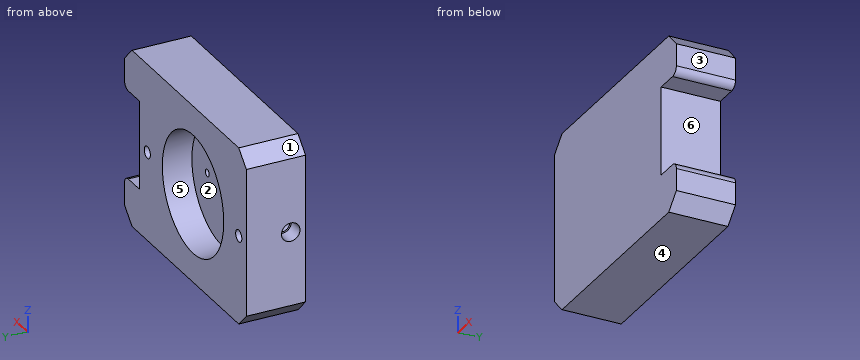
```python
from build123d import *

# Parameters (mm, degrees)
BOX_BODY_DEPTH                 = 25.4
SKETCH3_R                      = 25.5905
SAMPLE_HOLE_DEPTH              = 12.7
CUTOUT_EDGE_FILLET_R           = 3.175
BOX_EDGE_CHAMFER_SIZE          = 6.35
BOX_CLAMP_THREADED_HOLES_D     = 5.1054
BOX_CLAMP_THREADED_HOLES_DEPTH = 12.7
BOX_CLAMP_THREADED_HOLES_TIP   = 1.533816902
SKETCH10_R                     = 1.5875
CUT_EXTRUDE2_DEPTH             = 63.5
CUT_EXTRUDE3_REACH             = 14.7
FLUID_HOLES_R                  = 1.5875


with BuildPart() as part:
    # Sketch1 → box body (new body)
    with BuildSketch(Plane(origin=(0, 0, 0), x_dir=(1, 0, 0), z_dir=(0, 1, 0))):
        Polygon((-50.8, 38.1), (50.8, 38.1), (50.8, 19.05), (38.1, 19.05), (38.1, -19.05), (50.8, -19.05), (50.8, -38.1), (-50.8, -38.1), align=None)
    extrude(amount=BOX_BODY_DEPTH)

    # Sketch3 → sample hole (cut)
    with BuildSketch(Plane(origin=(0, 25.4, 0), x_dir=(1, 0, 0), z_dir=(0, 1, 0))):
        with Locations((-6.35, 0)):
            Circle(SKETCH3_R)
    extrude(amount=-SAMPLE_HOLE_DEPTH, mode=Mode.SUBTRACT)

    # cutout edge fillet
    cutout_edge_fillet_edges = [part.edges().sort_by_distance(p)[0] for p in [
        (50.8, 12.7, -19.05),
        (50.8, 12.7, 19.05),
    ]]
    fillet(cutout_edge_fillet_edges, radius=CUTOUT_EDGE_FILLET_R)

    # box edge chamfer
    box_edge_chamfer_edges = [part.edges().sort_by_distance(p)[0] for p in [
        (50.8, 12.7, 38.1),
        (-50.8, 12.7, 38.1),
        (-50.8, 12.7, -38.1),
        (50.8, 12.7, -38.1),
    ]]
    chamfer(box_edge_chamfer_edges, length=BOX_EDGE_CHAMFER_SIZE)

    # box clamp threaded holes
    with Locations(Plane(origin=(0, 25.4, 0), x_dir=(1, 0, 0), z_dir=(0, 1, 0))):
        with Locations((-44.45, 0), (31.75, 0)):
            Hole(BOX_CLAMP_THREADED_HOLES_D / 2, depth=BOX_CLAMP_THREADED_HOLES_DEPTH)
            with Locations((0, 0, -(BOX_CLAMP_THREADED_HOLES_DEPTH + BOX_CLAMP_THREADED_HOLES_TIP / 2))):  # 118° drill point
                Cone(0, BOX_CLAMP_THREADED_HOLES_D / 2, BOX_CLAMP_THREADED_HOLES_TIP, mode=Mode.SUBTRACT)

    # Sketch10 → Cut-Extrude2 (cut)
    with BuildSketch(Plane.ZY.offset(50.8)):
        with Locations((0, 6.35)):
            Circle(SKETCH10_R)
    extrude(amount=-CUT_EXTRUDE2_DEPTH, mode=Mode.SUBTRACT)

    # fluid holes → Cut-Extrude3 (cut, up to next)
    with BuildSketch(Plane(origin=(0, 12.7, 0), x_dir=(1, 0, 0), z_dir=(0, 1, 0)), mode=Mode.PRIVATE) as cut_extrude3_sk1:
        with Locations((-19.14525, 0)):
            Circle(FLUID_HOLES_R)
    cut_extrude3_tool1 = extrude(cut_extrude3_sk1.sketch, amount=-CUT_EXTRUDE3_REACH, mode=Mode.PRIVATE) & part.part
    add(cut_extrude3_tool1.solids().sort_by_distance((-19.14525, 12.7, 0))[0], mode=Mode.SUBTRACT)
    # fluid holes → Cut-Extrude3 (cut, up to next)
    with BuildSketch(Plane(origin=(0, 12.7, 0), x_dir=(1, 0, 0), z_dir=(0, 1, 0)), mode=Mode.PRIVATE) as cut_extrude3_sk2:
        with Locations((6.44525, 0)):
            Circle(FLUID_HOLES_R)
    cut_extrude3_tool2 = extrude(cut_extrude3_sk2.sketch, amount=-CUT_EXTRUDE3_REACH, mode=Mode.PRIVATE) & part.part
    add(cut_extrude3_tool2.solids().sort_by_distance((6.44525, 12.7, 0))[0], mode=Mode.SUBTRACT)

    # Sketch15 → 1/16 NPT Tapped Hole2 (revolve, cut)
    with BuildSketch(Plane(origin=(-50.8, 6.35, 0), x_dir=(0, 0, 1), z_dir=(0, 1, 0))):
        Polygon((0, 0), (0, 13.530685027), (3.0734, 11.684), (3.0734, 6.858), (3.762574096, 6.858), (3.9679118, 0), align=None)
    revolve(axis=Axis((-57.15, 6.35, 0), (1, 0, 0)), mode=Mode.SUBTRACT)


solid = part.part
```
Here's how the part is built. I have some questions about the finished solid (model axes, mm). Face numbers are marked on the shaded views. A direction names the side the tool comes from. Coordinates: 2 decimals unless noted, no trailing zeros. Loops run counter-clockwise (first coordinate to the right, second up) from the corner with the lowest first, then second, coordinate; pieces in that order, holes last. Notation, with made-up numbers: (27.25, 61.5) - (63.25, 61.5) arc R18 cw to (63.25, 79.5) - close; hole circle Ø5 at (19, 73). An arc over 180 degrees is marked (long way). Answer as CSV lines item,"result".
Q1. If we section it at C-C, the plane z = 10: Write out the boundary of the cut face in (x, y), and give its area (3 significant figures).
Response:
outline,"(-50.8, 0) - (38.1, 0) - (38.1, 25.4) - (17.21, 25.4) - (17.21, 12.7) - (-29.91, 12.7) - (-29.91, 25.4) - (-50.8, 25.4) - close"
area,"1,660 mm2"
Q2. For pin 1 (3.5 mm diameter, centred on y = 6.35, z = 0, fed in from -X); pin 2 (7.5 mm diameter, centred on y = 7.5, z = -7, fed in from +X); pin 3 (2.5 mm diameter, centred on y = 7.5, z = 0.5, fed in from -X), each with a flat end and sliding along its axis, tell me the tip position at first contact or that it passes through.
Response:
pin 1,"x = -38.32"
pin 2,"x = 38.1"
pin 3,"x = -38.77"
Q3. If I drill on L1, parallel to Z at x = 40.5, y = 11.5; L2, parallel to Z at x = -27.5, y = 6.25; L3, parallel to X at y = 8, z = 0, over which ranges is the centre line in solid material (lowest first)? Write a range as [from, to].
Response:
L1,"[-38.1, -19.05], [19.05, 38.1]"
L2,"[-38.1, -1.58], [1.58, 38.1]"
L3,"[-38.26, -20.73], [-17.56, 4.86], [8.03, 38.1]"
Q4. If we section it at D-D, the plane z = 33: Write out the boundary of the cut face in (x, y).
Response:
outline,"(-49.55, 0) - (49.55, 0) - (49.55, 25.4) - (-49.55, 25.4) - close"
Q5. We'd pull the mould along Z, two halves only. Please class the marked faces 1, 2 and 3: pulls with the +Z half, pulls with the -Z half, needs draft (parallel to the pull), parting line crosses it, or undercut.
Response:
face 1,"pulls with the +Z half"
face 2,"undercut"
face 3,"needs draft"
Q6. If we section it at A-A, the plane y = 20.5: Give the number of separate pieces and of enclosed holes in the cut face, and give its area (3 significant figures).
Response:
separate pieces,"1"
enclosed holes,"3"
area,"5,070 mm2"
Q7. For the marked faces 4, 5 and 6, which set-ups out of +Z, -Z, +X, -X, +Y, -Y let a thin tool reach every point of the face, with its end or its side?
Response:
face 4,"-Z, +X, -X, +Y, -Y"
face 5,"+Y"
face 6,"+X, +Y, -Y"
